Autodesk Inventor part; units mm, degrees
ref_plane "YZ Plane" through (0, 0, 0) normal (1, 0, 0) x (0, 1, 0)
ref_plane "XZ Plane" through (0, 0, 0) normal (0, 1, 0) x (-1, 0, 0)
ref_plane "XY Plane" through (0, 0, 0) normal (0, 0, 1) x (1, 0, 0)
sketch "Sketch1" plane through (0, 0, 0) normal (1, 0, 0) x (0, 1, 0)
  line L0 (-50, 110) -> (-50, -110)
  line L1 (-50, -110) -> (45, -110)
  line L2 (-50, 110) -> (-270, 110)
  line L3 (-270, 110) -> (-270, 280)
  line L4 (-270, 280) -> (70, 280)
  line L5 (70, -105) -> (-45, -105)
  line L6 (-45, -105) -> (-45, 115)
  line L7 (-45, 115) -> (-265, 115)
  line L8 (-265, 115) -> (-265, 275)
  line L9 (-265, 275) -> (45, 275)
  line L10 (-50, -110) -> (70, -110)
  line L11 (70, -110) -> (70, -105)
  line L12 (70, 275) -> (70, 280)
  line L13 (45, 275) -> (70, 275)
  point P0 (0, 0)
extrude "Extrusion1" add sketch "Sketch1" along normal blind 160
sketch "Sketch2" plane through (0, -45, 115) normal (0, 1, 0) x (1, 0, 0)
  circle A0 centre (80.342, 110) radius 7.5
  point P0 (0, 115)
  dimension "d10" = 15
extrude "Extrusion2" cut sketch "Sketch2" against normal blind 10
properties part number "Body Skeleton" material "Pine, Southern"
Build history of the part. All positions in model axes, mm. A direction names the side the tool comes from. Coordinates: 2 decimals unless noted, no trailing zeros. Order: outer loops, then holes, each group sorted by start corner. A loop starts at its lowest first (then second) coordinate and runs counter-clockwise, first axis right, second up. Notation, with made-up numbers: M 74.5,-15.75 L 113.5,-15.75 A23 cw 113.5,-7.75 Z; hole C 43,62 d6. An arc over 180 degrees is marked long. One line per question, with ' | ' between items. Start each with the question number.
Q1. Saw through at A-A (y = 22). List the corners of the cut face in (x, z).
Q2. Probe L1, parallel to Z at x = 114, y = -255; L2, parallel to X at y = -46.2, z = 5; L3, parallel to Z at x = 120, y = -40.5. List the from-to ranges inside material, lowest first. Write a range as from..to.
Q3. Saw through at C-C (x = 10). List the corners of the cut face in (y, z).
Q4. Flat gauge pins, fed straight in: pin 1 Ø6 at (x, z) = (26, 131) entering from +Y; pin 2 Ø1 at (x, y) = (64.5, -199.5) entering from -Z; pin 3 Ø24 at (x, z) = (80.342, 5) entering from -Y. Where does each tip first touch, or does it go through?
Q5. Two-plate mould, pull along Z, no slides. Class faces 1 (the face through (79, 9, -110)), 2 (the face through (0, -163.8, 114.8)), 3 (the face through (79, -153, 115)): +Z half, -Z half, draft (parallel to the pull), parting line (faces both ways), or undercut.
Q6. 3-axis set-ups, long thin cutter, end or side, ignore diameter. For faces 4 (the face through (97, -50, 2)), 5 (the face through (160, -163.8, 114.8)), 6 (the face through (97, -45, 3)): which of +Z, -Z, +X, -X, +Y, -Y reach the whole face in a straight line?
Q7. Saw through at D-D (z = 140.5). List the corners of the cut face in (x, y).
Q8. Saw through at B-B (z = 5). List the corners of the cut face in (x, y), then the cut area to 3 significant figures.
Check values:
1) outline: M 0,-110 L 160,-110 L 160,-105 L 0,-105 Z; M 0,275 L 160,275 L 160,280 L 0,280 Z
2) L1: z = 110..115, 275..280 | L2: x = 0..72.84, 87.84..160 | L3: z = -110..-105, 275..280
3) outline: M -270,110 L -50,110 L -50,-110 L 70,-110 L 70,-105 L -45,-105 L -45,115 L -265,115 L -265,275 L 70,275 L 70,280 L -270,280 Z
4) pin 1: stops at y = -265 | pin 2: stops at z = 110 | pin 3: stops at y = -50
5) face 1: -Z half | face 2: draft | face 3: undercut
6) face 4: -Z, +X, -X, -Y | face 5: +Z, -Z, +X, +Y, -Y | face 6: +X, -X, +Y
7) outline: M 0,-270 L 160,-270 L 160,-265 L 0,-265 Z
8) outline: M 0,-50 L 72.84,-50 L 72.84,-45 L 0,-45 Z; M 87.84,-50 L 160,-50 L 160,-45 L 87.84,-45 Z | area: 725 mm2
